Design review of the part shown in the three views and the two pictorial views. Dimensions are in mm from the part's minimum x, y and z. Coordinates: 2 decimals unless noted, no trailing zeros. Write each loop counter-clockwise with the first axis right and the second up, starting at its lowest first coordinate (ties: lowest second). Pieces come first, ordered by that corner, then holes. Notation, with made-up numbers: (-31, -24) -> (9, -24) arc R29 ccw to (9, 2) -> close; hole circle Ø9 at (2.5, 54.25). An arc over 180 degrees is marked (long way). Answer in a Markdown table with one row per item. Add a question column.
Item 1: Take a section at A-A, the plane x = 40. Write out the cut boundary in (y, z).
Item 2: Draft analysis for pull direction Z (two halves, no side actions). For the marked faces 1, 2, 3 and 4, state which applies: released by +Z, released by -Z, zero draft, split by the parting line, or undercut.
Item 3: Clearance check with flat-ended pins moving along their axes: P1, Ø1, axis at x = 37.5, y = 9.5, coming from the -Z side; P2, Ø4, axis at x = 40, z = 65, coming from the +Y side; P3, Ø5, axis at y = 2.5, z = 57, coming from the -X side. State where each tip first meets the part, or that it passes through.
Item 4: To check wall thickness, follow line 1 (Z direction, x = 40.5, y = 5.25); line 2 (X direction, y = 8.25, z = 40); line 3 (Z direction, x = 40, y = 1.55). State the ranges of each line that lie inside material, in increasing order.
Item 5: Take a section at D-D, the plane y = 9.25. Write out the cut boundary in (x, z), and give its area (3 significant figures).
Item 6: Take a section at C-C, the plane y = 2.5. Write out the cut boundary in (x, z), and give its area (3 significant figures).
Item 7: Take a section at B-B, the plane z = 40. Write out the cut boundary in (x, y), and give its area (3 significant figures).
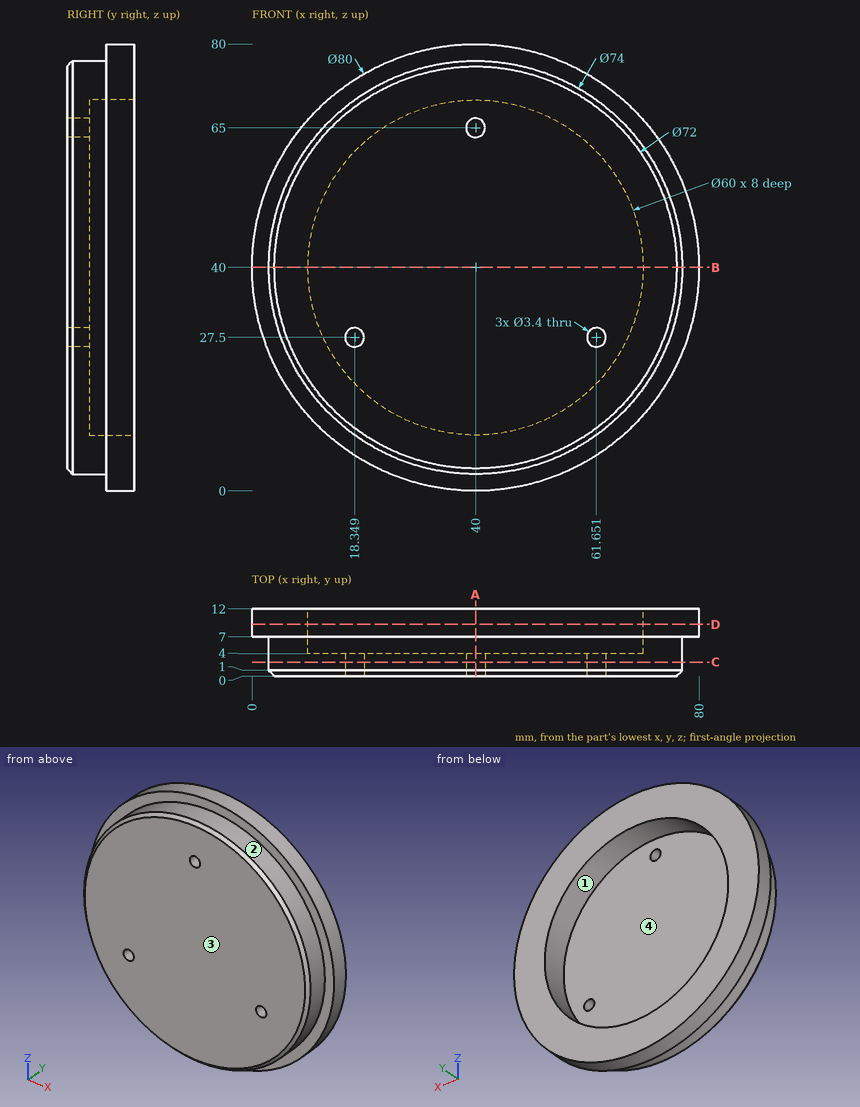
Answers:
| question | item | result |
|---|---|---|
| 1 | outline | (0, 4) -> (1, 3) -> (7, 3) -> (7, 0) -> (12, 0) -> (12, 10) -> (4, 10) -> (4, 63.3) -> (0, 63.3) -> close; (0, 66.7) -> (4, 66.7) -> (4, 70) -> (12, 70) -> (12, 80) -> (7, 80) -> (7, 77) -> (1, 77) -> (0, 76) -> close |
| 2 | face 1 | undercut |
| 2 | face 2 | split by the parting line |
| 2 | face 3 | zero draft |
| 2 | face 4 | undercut |
| 3 | P1 | stops at z = 0.05 |
| 3 | P2 | stops at y = 4 |
| 3 | P3 | stops at x = 5.96 |
| 4 | line 1 | z = 3 to 10, 70 to 77 |
| 4 | line 2 | x = 0 to 10, 70 to 80 |
| 4 | line 3 | z = 3 to 63.3, 66.7 to 77 |
| 5 | outline | circle Ø80 at (40, 40); hole circle Ø60 at (40, 40) |
| 5 | area | 2,200 mm^2 |
| 6 | outline | circle Ø74 at (40, 40); hole circle Ø3.4 at (18.35, 27.5); hole circle Ø3.4 at (40, 65); hole circle Ø3.4 at (61.65, 27.5) |
| 6 | area | 4,270 mm^2 |
| 7 | outline | (0, 7) -> (3, 7) -> (3, 1) -> (4, 0) -> (76, 0) -> (77, 1) -> (77, 7) -> (80, 7) -> (80, 12) -> (70, 12) -> (70, 4) -> (10, 4) -> (10, 12) -> (0, 12) -> close |
| 7 | area | 437 mm^2 |
